Here's how the part is built. I have some questions about the finished solid (model axes, mm). Face numbers are marked on the shaded views. A direction names the side the tool comes from. Coordinates: 2 decimals unless noted, no trailing zeros. Write each loop counter-clockwise with the first axis right and the second up, starting at its lowest first coordinate (ties: lowest second). Pieces come first, ordered by that corner, then holes.
```python
from build123d import *

# Parameters (mm, degrees)
F2_SIZE = 0.25


with BuildPart() as f1:
    # F0 (on Front) → F1 (revolve)
    with BuildSketch(Plane.XZ):
        Polygon((-19, 0), (0, 0), (0, 5), (-10, 5), (-10, 3), (-16.5, 3), (-16.5, 2.85), (-17.3, 2.85), (-17.3, 3), (-19, 3), align=None)
    revolve(axis=Axis((6.458773, 0, 0), (1, 0, 0)))

    # F2
    f2_edges = [f1.edges().sort_by_distance(p)[0] for p in [
        (0, 0, -5),
        (-10, 0, -5),
        (-5, 0, 5),
        (-19, 0, -3),
    ]]
    chamfer(f2_edges, length=F2_SIZE)


solid = f1.part
```
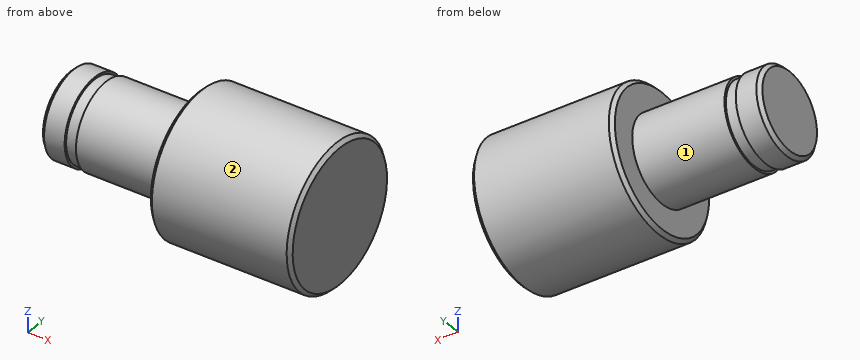
1) Will these pins go through, and if not, where does the flat tip stop? pin 1 (3 mm diameter, centred on x = -8, y = 3, fed in from +Z); pin 2 (4 mm diameter, centred on x = -7.5, z = 4, fed in from -Y); pin 3 (4 mm diameter, centred on x = -12.5, z = 3, fed in from -Y).
Values follow:
pin 1: stops at z = 4.77
pin 2: stops at y = -4.58
pin 3: stops at y = -2.83
2) On a 3-axis mill with a long thin cutter (end or side, diameter ignored), from which of +Z, -Z, +X, -X, +Y, -Y can I reach the whole of each face in a straight line? I mean the marked faces 1 and 2. Say none if no direction works.
Values follow:
face 1: -X
face 2: +X, -X
3) Imagine slicing it at D-D on x = -12.5. Please give me the cut outline in (y, z), then the cut area to 3 significant figures.
Values follow:
outline: circle Ø6 at (0, 0)
area: 28.3 mm2
4) Imagine slicing it at C-C on x = -17. Please give me the cut outline in (y, z).
Values follow:
outline: circle Ø5.7 at (0, 0)
5) I need wall thicknesses on probe 1 along X at (y, z) = (3.25, 2.5); probe 2 along Z at (x, y) = (-17, 0); probe 3 along Z at (x, y) = (-17.5, -0.75). Which ranges of each line are inside material? Lowest first, please.
Values follow:
probe 1: x = -10 to 0
probe 2: z = -2.85 to 2.85
probe 3: z = -2.9 to 2.9
6) Imagine slicing it at A-A on z = 0. Please give me the cut outline in (x, y), then the cut area to 3 significant figures.
Values follow:
outline: (-19, -2.75) - (-18.75, -3) - (-17.3, -3) - (-17.3, -2.85) - (-16.5, -2.85) - (-16.5, -3) - (-10, -3) - (-10, -4.75) - (-9.75, -5) - (-0.25, -5) - (0, -4.75) - (0, 4.75) - (-0.25, 5) - (-9.75, 5) - (-10, 4.75) - (-10, 3) - (-16.5, 3) - (-16.5, 2.85) - (-17.3, 2.85) - (-17.3, 3) - (-18.75, 3) - (-19, 2.75) - close
area: 154 mm2
